Verification items for the finished model (mm, model axes). A direction names the side the tool comes from. Round coordinates to 2 decimals unless told otherwise and drop trailing zeros. Loops run counter-clockwise (first coordinate to the right, second up) from the corner with the lowest first, then second, coordinate; pieces in that order, holes last. Notation, with made-up numbers: (18.25, 72.25) -> (39.25, 72.25) arc R24 ccw to (39.25, 101.25) -> close; hole circle Ø8 at (17, -38.5). An arc over 180 degrees is marked (long way). Write item = value, one per line.
```python
from build123d import *

# Parameters (mm, degrees)
CHAMFER_1_SIZE      = 0.3
SKETCH_2_OUTSIDE_W  = 18.352
SKETCH_2_OUTSIDE_H  = 18.352
CUT_EXTRUDE_1_DEPTH = 15.495689014


with BuildPart() as part:
    # Sketch 1 → Revolve 1 (revolve)
    with BuildSketch(Plane.XY, mode=Mode.PRIVATE) as revolve_1_sk:
        Polygon((1.5, 0), (4, 0), (4, -4.5), (3.25, -4.5), (3.25, -6), (5.75, -6), (5.75, -10), (3.682615316, -10), (2.75, -12), (2.75, -18), (1.5, -18), align=None)
    revolve(revolve_1_sk.sketch.rotate(Axis((0, 8.266911596, 0), (0, -1, 0)), 90), axis=Axis((0, 8.266911596, 0), (0, -1, 0)))

    # Chamfer 1
    chamfer_1_edges = [part.edges().sort_by_distance(p)[0] for p in [
        (0, -6, -5.75),
        (0, -4.5, -4),
        (0, 0, -4),
        (0, -18, -1.5),
        (0, -18, -2.75),
        (0, -10, -5.75),
    ]]
    chamfer(chamfer_1_edges, length=CHAMFER_1_SIZE)

    # Sketch 2 outside → Cut-Extrude 1 (cut, through all)
    with BuildSketch(Plane(origin=(0, -6, 0), x_dir=(1, 0, 0), z_dir=(0, 1, 0))):
        Rectangle(SKETCH_2_OUTSIDE_W, SKETCH_2_OUTSIDE_H)
        Polygon((5.773502692, 0), (2.886751346, 5), (-2.886751346, 5), (-5.773502692, 0), (-2.886751346, -5), (2.886751346, -5), align=None, mode=Mode.SUBTRACT)
    extrude(amount=-CUT_EXTRUDE_1_DEPTH, mode=Mode.SUBTRACT)


solid = part.part
```
(1) Sectioned sample at C-C, the plane y = -2.5. Record the cut outline in (x, z), and give its area (3 significant figures).
Filled sheet:
outline = circle Ø8 at (0, 0); hole circle Ø3 at (0, 0)
area = 43.2 mm2
(2) Go/stop test with flat-tipped pins: pin 1 Ø1.5 at (x, z) = (-1.5, 2) entering from +Y; pin 2 Ø4 at (y, z) = (-14.5, 3.5) entering from -X. Record where each tip stops, or that it passes through.
Filled sheet:
pin_1 = 0
pin_2 = -2.3
(3) Material ranges on probe 1 along X at (y, z) = (-8, 0); probe 2 along Y at (x, z) = (4, -1.25); probe 3 along X at (y, z) = (-10.75, 0), recorded low to high. Write a range as from..to.
Filled sheet:
probe_1 = -5.75..-1.5, 1.5..5.75
probe_2 = -10..-6
probe_3 = -3.33..-1.5, 1.5..3.33
(4) Sectioned sample at D-D, the plane y = -10.25. Record the cut outline in (x, z), and give its area (3 significant figures).
Filled sheet:
outline = circle Ø7.13 at (0, 0); hole circle Ø3 at (0, 0)
area = 32.9 mm2
(5) Set-up check for faces 4 (the face through (3.905, -2.277, -0.867)), 5 (the face through (-4, -10, 0)), 6 (the face through (-0.1, -6, 3.4)): record each of +Z, -Z, +X, -X, +Y, -Y from which the full face is reachable in a straight line by a thin tool's end or side.
Filled sheet:
face_4 = +Y
face_5 = -Y
face_6 = none
(6) Draft check along X on faces 1 (the face through (0, -8, -5)), 2 (the face through (-4.35, -7.972, 2.466)), 3 (the face through (-0.45, -8.73, 1.43)). Enter one of: released by +X, released by -X, zero draft, split by the parting line, or undercut.
Filled sheet:
face_1 = zero draft
face_2 = released by -X
face_3 = undercut
(7) Sectioned sample at B-B, the plane y = -7.5. Record the cut outline in (x, z), and give its area (3 significant figures).
Filled sheet:
outline = (-5.75, -0.04) -> (-2.91, -4.96) arc R5.75 ccw to (-2.84, -5) -> (2.84, -5) arc R5.75 ccw to (2.91, -4.96) -> (5.75, -0.04) arc R5.75 ccw to (5.75, 0.04) -> (2.91, 4.96) arc R5.75 ccw to (2.84, 5) -> (-2.84, 5) arc R5.75 ccw to (-2.91, 4.96) -> (-5.75, 0.04) arc R5.75 ccw to start; hole circle Ø3 at (0, 0)
area = 79.5 mm2
